The model under review builds one solid part; all positions refer to its coordinate system, in mm. A direction names the side the tool comes from. Round coordinates to 2 decimals unless told otherwise and drop trailing zeros. Order: outer loops, then holes, each group sorted by start corner. A loop starts at its lowest first (then second) coordinate and runs counter-clockwise, first axis right, second up. Notation, with made-up numbers: (78, -25.75) -> (108, -25.75) arc R20 cw to (108, 10.25) -> close; hole circle Ø4 at (-27.5, -20). An arc over 180 degrees is marked (long way). Return JSON: item names as keys, results as strings. Group by question number.
from build123d import *

# Parameters (mm, degrees)
F0_W = 14.6103731854
F0_H = 11.8872


# Not quite as in the source:
# - ends of sketch curves that miss each other by under 0.0002 mm in the source are joined


with BuildPart() as f1:
    # F0 (on Front) → F1 (revolve)
    with BuildSketch(Plane.XZ):
        with Locations((-13.6665977984, 5.9436)):
            Rectangle(F0_W, F0_H)
        with BuildLine():
            Line((-6.3614112057, 11.8872), (-6.3614112057, 0))
            Line((-6.3614112057, 0), (15.6496424236, 0))
            Line((15.6496424236, 0), (15.6496424236, 11.8872))
            Line((15.6496424236, 11.8872), (15.6496424236, 25.9283669293))
            Line((15.6496424236, 25.9283669293), (14.1691156089, 22.7533669293))
            ThreePointArc((14.1691156089, 22.7533669293), (11.3793089407, 16.0181760794), (4.6441191189, 13.2283669293))
            ThreePointArc((4.6441191189, 13.2283669293), (-2.0910777228, 16.0181760794), (-4.8808843911, 22.7533669293))
            Line((-4.8808843911, 22.7533669293), (-6.3614112057, 25.9283669293))
            Line((-6.3614112057, 25.9283669293), (-6.3614112057, 11.8872))
        make_face()
        with Locations((22.9548290163, 5.9436)):
            Rectangle(F0_W, F0_H)
    revolve(axis=Axis((4.6441156089, 0, 0), (1, 0, 0)))


solid = f1.part
Item 1: Wall thickness on line 1 along X through (y, z) = (-5.5, -11); line 2 along Y through (x, z) = (19, 0); line 3 along X through (y, z) = (1.5, 21.5): over which ranges is each line inside the solid? List them lowest first.
Item 2: Consider section A-A on x = 20.5. State the section outline as (y, z) points, plus the area to 3 significant figures.
Item 3: Insertion check: pin 1 Ø5 at (y, z) = (1, 16.5) entering from -X; pin 2 Ø3 at (x, y) = (18.5, -10.5) entering from -Z; pin 3 Ø10 at (x, z) = (-0.5, 11.5) entering from -Y. Each pin has a flat end and moves straight along its axis. Give the tip position at first contact, or say it passes through.
Item 4: Consider section B-B on x = 10.5. State the section outline as (y, z) points.
Item 5: For faces 4 (the face through (-6.361, 5, 11)), 5 (the face through (-4.97, -6.89, 21.89)), 6 (the face through (15.65, 5, -11)), 7 (the face through (30.26, 0, 0)), list the 3-axis set-ups (+Z, -Z, +X, -X, +Y, -Y) from which the entire face can be reached by the end or side of a thin tool; tool diameter is ignored.
Item 6: The part is to be moulded in two halves that separate along X. For faces 1 (the face through (-20.972, 0, 0)), 2 (the face through (14.24, -6.88, 21.85)), 3 (the face through (23.06, -3.57, 11.34)), say which applies: +X half, -X half, draft (parallel to the pull), parting line (faces both ways), or undercut.
Values:
{
 "1": {"line 1": "-6.36 to 15.65", "line 2": "-11.89 to 11.89", "line 3": "-6.36 to -4.8, 14.09 to 15.65"},
 "2": {"outline": "circle Ø23.77 at (0, 0)", "area": "444 mm^2"},
 "3": {"pin 1": "x = -6.36", "pin 2": "z = -7.77", "pin 3": "y = -21.43"},
 "4": {"outline": "circle Ø30.48 at (0, 0)"},
 "5": {"face 4": "-X", "face 5": "none", "face 6": "+X", "face 7": "+Z, -Z, +X, +Y, -Y"},
 "6": {"face 1": "-X half", "face 2": "undercut", "face 3": "draft"}
}
